Work out the finished part from the listing and answer in its coordinate system (mm). A direction names the side the tool comes from. Coordinates: 2 decimals unless noted, no trailing zeros. Write each loop counter-clockwise with the first axis right and the second up, starting at its lowest first coordinate (ties: lowest second). Pieces come first, ordered by that corner, then holes. Notation, with made-up numbers: (2, 33.25) - (20, 33.25) arc R28 ccw to (20, 58.25) - close; hole circle Ø6 at (38, 16.5). An arc over 180 degrees is marked (long way). Use a Markdown table: item, result. Add a question column.
(1) The part is cut by section C-C, the plane z = -23. Give the vertices of the cut face in (x, y).
(2) The part is cut by section B-B, the plane y = 79.5. Give the vertices of the cut face in (x, z).
(3) The part is cut by section A-A, the plane x = -3. Give the vertices of the cut face in (y, z), then the cut area to 4 significant figures.
(4) A tool of negligible diameter and unlimited length cuts with its end or side. For faces 4 (the face through (-16.239, 230.594, 3.719)), 5 (the face through (0, 228.2, -31)), 6 (the face through (1, 220, -6)), from which of +Z, -Z, +X, -X, +Y, -Y can it reach the whole face along a straight path? Write none if from no direction.
(5) The part is cut by section D-D, the plane z = -14. Give the vertices of the cut face in (x, y), then the cut area to 3 significant figures.
(6) Given pin 1 Ø1.3 at (x, z) = (-16.5, -41) entering from -Y; pin 2 Ø1.3 at (x, y) = (16, 73.5) entering from -Z; pin 3 Ø6 at (y, z) = (220, -7) entering from -X, each flat-ended and moving along its own axis, determine where each tip first touches the part or whether it passes through.
(7) For a pull along X with two mould halves and no side action, classify faces 1 (the face through (-12.25, 228.81, 1.9)), 2 (the face through (-1, 220, -6)), 3 (the face through (16.24, 231.43, 4.58)) as released by +X, released by -X, zero draft, split by the parting line, or undercut.
(8) Find the intervals of material crossed by line 1 (Z direction, x = 15, y = 92); line 2 (Y direction, x = -6, z = -51.5); line 3 (Z direction, x = -8, y = 166), in increasing order. Write a range as from..to.
from build123d import *

# Parameters (mm, degrees)
RIB_3_REACH     = 244.396
SKETCH_3_WALL_W = 515.076556858
SKETCH_3_WALL_H = 2


with BuildPart() as part:
    # 扫描1: sweep along a path in 草图2
    with BuildLine(Plane(origin=(0, 0, 0), x_dir=(0, 0, -1), z_dir=(1, 0, 0))) as sweep_1_path:
        Line((0, 0), (0, 225))
        ThreePointArc((0, 225), (0.585786438, 226.414213562), (2, 227))
        Line((2, 227), (60, 227))
    # 草图1 → 扫描1 (sweep)
    with BuildSketch(Plane(origin=(0, 0, 0), x_dir=(1, 0, 0), z_dir=(0, 1, 0))):
        with BuildLine():
            Line((17.5, -7.2), (14.94151844, -7.2))
            ThreePointArc((14.94151844, -7.2), (13.772097871, -6.82248437), (13.044151844, -5.832455532))
            Line((13.044151844, -5.832455532), (11.955848156, -2.567544468))
            ThreePointArc((11.955848156, -2.567544468), (11.227902129, -1.57751563), (10.05848156, -1.2))
            Line((10.05848156, -1.2), (-10.05848156, -1.2))
            ThreePointArc((-10.05848156, -1.2), (-11.227902129, -1.57751563), (-11.955848156, -2.567544468))
            Line((-11.955848156, -2.567544468), (-13.044151844, -5.832455532))
            ThreePointArc((-13.044151844, -5.832455532), (-13.772097871, -6.82248437), (-14.94151844, -7.2))
            Line((-14.94151844, -7.2), (-17.5, -7.2))
            Line((-17.5, -7.2), (-17.5, -6))
            Line((-17.5, -6), (-14.94151844, -6))
            ThreePointArc((-14.94151844, -6), (-14.473750212, -5.848993748), (-14.182571802, -5.452982213))
            Line((-14.182571802, -5.452982213), (-13.094268114, -2.188071149))
            ThreePointArc((-13.094268114, -2.188071149), (-11.929554471, -0.604025007), (-10.05848156, 0))
            Line((-10.05848156, 0), (10.05848156, 0))
            ThreePointArc((10.05848156, 0), (11.929554471, -0.604025007), (13.094268114, -2.188071149))
            Line((13.094268114, -2.188071149), (14.182571802, -5.452982213))
            ThreePointArc((14.182571802, -5.452982213), (14.473750212, -5.848993748), (14.94151844, -6))
            Line((14.94151844, -6), (17.5, -6))
            Line((17.5, -6), (17.5, -7.2))
        make_face()
    sweep(path=sweep_1_path.line)

    # 草图3 wall → 筋3 (add, up to next)
    with BuildSketch(Plane(origin=(0, 217, -10), x_dir=(0, 0.707106781187, -0.707106781187), z_dir=(0, 0.707106781187, 0.707106781187)), mode=Mode.PRIVATE) as rib_3_sk1:
        Rectangle(SKETCH_3_WALL_W, SKETCH_3_WALL_H)
    rib_3_tool1 = extrude(rib_3_sk1.sketch, amount=RIB_3_REACH, mode=Mode.PRIVATE) - part.part
    add(rib_3_tool1.solids().sort_by_distance((0, 217, -10))[0])


solid = part.part
Model answer:
| question | item | result |
|---|---|---|
| 1 | outline | (-17.5, 233) - (-14.94, 233) arc R0.8 cw to (-14.18, 232.45) - (-13.09, 229.19) arc R3.2 ccw to (-10.06, 227) - (10.06, 227) arc R3.2 ccw to (13.09, 229.19) - (14.18, 232.45) arc R0.8 cw to (14.94, 233) - (17.5, 233) - (17.5, 234.2) - (14.94, 234.2) arc R2 ccw to (13.04, 232.83) - (11.96, 229.57) arc R2 cw to (10.06, 228.2) - (-10.06, 228.2) arc R2 cw to (-11.96, 229.57) - (-13.04, 232.83) arc R2 ccw to (-14.94, 234.2) - (-17.5, 234.2) - close |
| 2 | outline | (-17.5, 6) - (-14.94, 6) arc R0.8 cw to (-14.18, 5.45) - (-13.09, 2.19) arc R3.2 ccw to (-10.06, 0) - (10.06, 0) arc R3.2 ccw to (13.09, 2.19) - (14.18, 5.45) arc R0.8 cw to (14.94, 6) - (17.5, 6) - (17.5, 7.2) - (14.94, 7.2) arc R2 ccw to (13.04, 5.83) - (11.96, 2.57) arc R2 cw to (10.06, 1.2) - (-10.06, 1.2) arc R2 cw to (-11.96, 2.57) - (-13.04, 5.83) arc R2 ccw to (-14.94, 7.2) - (-17.5, 7.2) - close |
| 3 | outline | (0, 0) - (225, 0) arc R2 cw to (227, -2) - (227, -60) - (228.2, -60) - (228.2, -2) arc R3.2 ccw to (225, 1.2) - (0, 1.2) - close |
| 3 | area | 344.5 mm^2 |
| 4 | face 4 | -Z, -X, -Y |
| 4 | face 5 | +Z, -Z, +Y |
| 4 | face 6 | -Z, +X, -Y |
| 5 | outline | (-17.5, 233) - (-14.94, 233) arc R0.8 cw to (-14.18, 232.45) - (-13.09, 229.19) arc R3.2 ccw to (-10.06, 227) - (-1, 227) - (-1, 221) - (1, 221) - (1, 227) - (10.06, 227) arc R3.2 ccw to (13.09, 229.19) - (14.18, 232.45) arc R0.8 cw to (14.94, 233) - (17.5, 233) - (17.5, 234.2) - (14.94, 234.2) arc R2 ccw to (13.04, 232.83) - (11.96, 229.57) arc R2 cw to (10.06, 228.2) - (-10.06, 228.2) arc R2 cw to (-11.96, 229.57) - (-13.04, 232.83) arc R2 ccw to (-14.94, 234.2) - (-17.5, 234.2) - close |
| 5 | area | 62.5 mm^2 |
| 6 | pin 1 | y = 233 |
| 6 | pin 2 | z = 6 |
| 6 | pin 3 | x = -1 |
| 7 | face 1 | undercut |
| 7 | face 2 | released by -X |
| 7 | face 3 | zero draft |
| 8 | line 1 | 6..7.2 |
| 8 | line 2 | 227..228.2 |
| 8 | line 3 | 0..1.2 |
